Here's how the part is built. I have some questions about the finished solid (model axes, mm). Face numbers are marked on the shaded views. A direction names the side the tool comes from. Round coordinates to 2 decimals unless told otherwise and drop trailing zeros. Write each loop counter-clockwise with the first axis right and the second up, starting at its lowest first coordinate (ties: lowest second). Pieces come first, ordered by that corner, then holes. Notation, with made-up numbers: (69.5, 47) - (100.5, 47) arc R10 cw to (100.5, 64) - close; hole circle Ø6 at (25.25, 84.25). An arc over 180 degrees is marked (long way). Write item = value, one per line. Start each with the question number.
Item 1: For P1, Ø2, axis at x = -43.5, y = 3, coming from the -Z side; P2, Ø2, axis at y = 2.5, z = -10, coming from the +X side; P3, Ø16.5, axis at x = -25, z = -8.5, coming from the +Y side, each with a flat end and sliding along its axis, tell me the tip position at first contact or that it passes through.
Item 2: Thinking about a two-plate mould opening in Z: for the marked faces 3 and 4, which applies, pulls with the +Z half, pulls with the -Z half, needs draft (parallel to the pull), parting line crosses it, or undercut?
Item 3: If we section it at A-A (x = 36.5): Please give me the cut outline in (y, z).
Item 4: If we section it at B-B (z = -7.5): Please give me the cut outline in (x, y), and give its area (3 significant figures).
Item 5: Which directions (+Z, -Z, +X, -X, +Y, -Y) give clear straight access to the entire face, cutting with the end or side of a thin tool? Please do the marked faces 1 and 2.
Item 6: If I drill on line 1 along X through (y, z) = (2.1, 16.5); line 2 along X through (y, z) = (0.6, 5); line 3 along Z through (x, y) = (7.5, 3.9), over which ranges is the centre line in solid material (lowest first)? Write a range as [from, to].
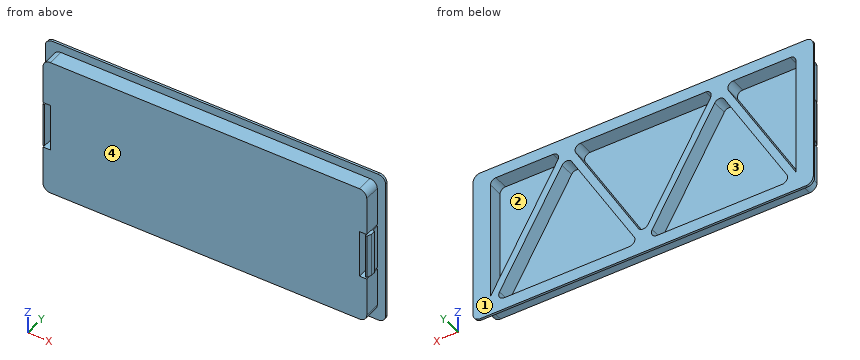
```python
from build123d import *

# Parameters (mm, degrees)
SKETCH1_W           = 88.1
SKETCH1_H           = 38.1
BOSS_EXTRUDE1_DEPTH = 5
SHELL1_T            = -1
SKETCH2_W           = 92.6
SKETCH2_H           = 42.6
SKETCH2_W_2         = 88.1
SKETCH2_H_2         = 38.1
BOSS_EXTRUDE2_DEPTH = 0.6
SKETCH5_W           = 2.5
SKETCH5_H           = 38.1
BOSS_EXTRUDE4_DEPTH = 5
SKETCH7_W           = 2
SKETCH7_H           = 13.01498231
CUT_EXTRUDE2_DEPTH  = 4.4
SKETCH8_W           = 0.4
SKETCH8_H           = 12.02996462
BOSS_EXTRUDE5_DEPTH = 4.4
BOSS_EXTRUDE6_DEPTH = 12.02996462
BOSS_EXTRUDE3_DEPTH = 4
SKETCH4_W           = 88.1
SKETCH4_H           = 100
CUT_EXTRUDE1_DEPTH  = 4.4
FILLET1_R           = 2
FILLET2_R           = 1.5


with BuildPart() as part:
    # Sketch1 → Boss-Extrude1 (new body)
    with BuildSketch(Plane(origin=(0, 0, 0), x_dir=(1, 0, 0), z_dir=(0, 1, 0))):
        Rectangle(SKETCH1_W, SKETCH1_H)
    extrude(amount=BOSS_EXTRUDE1_DEPTH)

    # Shell1
    shell1_openings = [part.faces().sort_by_distance(p)[0] for p in [
        (0, 5, 0),
    ]]
    offset(amount=SHELL1_T, openings=shell1_openings, kind=Kind.INTERSECTION)

    # Sketch2 → Boss-Extrude2 (add)
    with BuildSketch(Plane(origin=(0, 5, 0), x_dir=(1, 0, 0), z_dir=(0, 1, 0))):
        Rectangle(SKETCH2_W, SKETCH2_H)
        Rectangle(SKETCH2_W_2, SKETCH2_H_2, mode=Mode.SUBTRACT)
    extrude(amount=-BOSS_EXTRUDE2_DEPTH)

    # Sketch5 → Boss-Extrude4 (add)
    with BuildSketch(Plane.XZ):
        with Locations((42.8, 0)):
            Rectangle(SKETCH5_W, SKETCH5_H)
    boss_extrude4 = extrude(amount=-BOSS_EXTRUDE4_DEPTH)

    # Sketch7 → Cut-Extrude2 (cut)
    with BuildSketch(Plane.XZ):
        with Locations((43.05, 0.007491155)):
            Rectangle(SKETCH7_W, SKETCH7_H)
    cut_extrude2 = extrude(amount=-CUT_EXTRUDE2_DEPTH, mode=Mode.SUBTRACT)

    # Sketch8 → Boss-Extrude5 (add)
    with BuildSketch(Plane.XZ.offset(-4.4)):
        with Locations((43.85, 0)):
            Rectangle(SKETCH8_W, SKETCH8_H)
    boss_extrude5 = extrude(amount=BOSS_EXTRUDE5_DEPTH)

    # Sketch9 → Boss-Extrude6 (add)
    with BuildSketch(Plane(origin=(0, 0, -6.01498231), x_dir=(-1, 0, 0), z_dir=(0, 0, -1))):
        Polygon((-44.05, 0), (-44.55, 1.237543427), (-44.55, 2.5), (-44.05, 2.5), align=None)
    boss_extrude6 = extrude(amount=-BOSS_EXTRUDE6_DEPTH)

    # Mirror1: Boss-Extrude4, Cut-Extrude2, Boss-Extrude5, Boss-Extrude6 across plane
    add(boss_extrude4.mirror(Plane(origin=(0, 0, 0), x_dir=(0, 0, 1), z_dir=(1, 0, 0))))
    add(cut_extrude2.mirror(Plane(origin=(0, 0, 0), x_dir=(0, 0, 1), z_dir=(1, 0, 0))), mode=Mode.SUBTRACT)
    add(boss_extrude5.mirror(Plane(origin=(0, 0, 0), x_dir=(0, 0, 1), z_dir=(1, 0, 0))))
    add(boss_extrude6.mirror(Plane(origin=(0, 0, 0), x_dir=(0, 0, 1), z_dir=(1, 0, 0))))

    # Sketch3 → Boss-Extrude3 (add)
    with BuildSketch(Plane(origin=(0, 5, 0), x_dir=(1, 0, 0), z_dir=(0, 1, 0))):
        Polygon((-42.416724684, 17.551213149), (-20.775, -20.0548644), (0, 16.0451356), (20.775, -20.0548644), (42.416724684, 17.551213149), (40.683275316, 18.548786851), (20.775, -16.0451356), (0, 20.0548644), (-20.775, -16.0451356), (-40.683275316, 18.548786851), align=None)
    extrude(amount=-BOSS_EXTRUDE3_DEPTH)

    # Sketch4 → Cut-Extrude1 (cut)
    with BuildSketch(Plane.XZ):
        with Locations((0, 69.05)):
            Rectangle(SKETCH4_W, SKETCH4_H)
        with Locations((0, -69.05)):
            Rectangle(SKETCH4_W, SKETCH4_H)
    extrude(amount=-CUT_EXTRUDE1_DEPTH, mode=Mode.SUBTRACT)

    # Fillet1
    fillet1_edges = [part.edges().sort_by_distance(p)[0] for p in [
        (-44.05, 2.2, -19.05),
        (44.05, 2.2, -19.05),
        (44.05, 2.2, 19.05),
        (-44.05, 2.2, 19.05),
        (-46.3, 4.7, -21.3),
        (46.3, 4.7, -21.3),
        (46.3, 4.7, 21.3),
        (-46.3, 4.7, 21.3),
    ]]
    fillet(fillet1_edges, radius=FILLET1_R)

    # Fillet2
    fillet2_edges = [part.edges().sort_by_distance(p)[0] for p in [
        (-41.55, 3, 18.05),
        (-21.928768917, 3, 18.05),
        (-40.396231083, 3, -18.05),
        (-1.153768917, 3, -18.05),
        (-20.775, 3, 16.0451356),
        (1.153768917, 3, -18.05),
        (40.396231083, 3, -18.05),
        (20.775, 3, 16.0451356),
        (21.928768917, 3, 18.05),
        (19.621231083, 3, 18.05),
        (-19.621231083, 3, 18.05),
        (0, 3, -16.0451356),
        (41.55, 3, 18.05),
    ]]
    fillet(fillet2_edges, radius=FILLET2_R)


solid = part.part
```
Reply:
q1.P1 = -19
q1.P2 = 44.05
q1.P3 = 1
q2.face_3 = undercut
q2.face_4 = needs draft
q3.outline = (0, -19.05) - (4.4, -19.05) - (4.4, -21.3) - (5, -21.3) - (5, -18.05) - (1, -18.05) - (1, -11.28) - (5, -11.28) - (5, -7.27) - (1, -7.27) - (1, 18.05) - (5, 18.05) - (5, 21.3) - (4.4, 21.3) - (4.4, 19.05) - (0, 19.05) - close
q4.outline = (-46.3, 4.4) - (-44.05, 4.4) - (-44.05, 0) - (44.05, 0) - (44.05, 4.4) - (46.3, 4.4) - (46.3, 5) - (41.55, 5) - (41.55, 1) - (36.63, 1) - (36.63, 5) - (34.32, 5) - (34.32, 1) - (7.23, 1) - (7.23, 5) - (4.92, 5) - (4.92, 1) - (-4.92, 1) - (-4.92, 5) - (-7.23, 5) - (-7.23, 1) - (-34.32, 1) - (-34.32, 5) - (-36.63, 5) - (-36.63, 1) - (-41.55, 1) - (-41.55, 5) - (-46.3, 5) - close
q4.area = 148 mm2
q5.face_1 = +Z, -Z, +X, -X, +Y
q5.face_2 = +Y
q6.line_1 = [-44.05, -41.55], [-23.02, -18.53], [18.53, 23.02], [41.55, 44.05]
q6.line_2 = [-44.29, -43.65], [-42.05, 42.05], [43.65, 44.29]
q6.line_3 = [-19.05, -18.05], [-7.02, -3.01], [18.05, 19.05]
